```python
from build123d import *

# Parameters (mm, degrees)
SKETCH2_W                = 100
SKETCH2_H                = 100
BOSS_EXTRUDE1_DEPTH      = 5
SKETCH3_R                = 19.95
BOSS_EXTRUDE2_DEPTH      = 60
SKETCH4_R                = 5
CUT_EXTRUDE1_DEPTH       = 43.5
SKETCH10_R               = 1
SKETCH11_R               = 1
SKETCH15_R               = 5
BOSS_EXTRUDE3_DEPTH      = 10
BOSS_EXTRUDE3_DEPTH_BACK = 2
SKETCH18_R               = 5
BOSS_EXTRUDE4_DEPTH      = 1
SKETCH19_R               = 2.7
CUT_EXTRUDE3_DEPTH       = 36
SKETCH20_R               = 0.75
CUT_REVOLVE4_ANGLE       = 180
SKETCH21_W               = 20
SKETCH21_H               = 20
CUT_EXTRUDE4_DEPTH       = 2
SKETCH23_R               = 1.5
BOSS_EXTRUDE5_DEPTH      = 5


with BuildPart() as part:
    # Sketch2 → Boss-Extrude1 (new body)
    with BuildSketch(Plane(origin=(0, 0, 0), x_dir=(1, 0, 0), z_dir=(0, 1, 0))):
        with Locations((-25, 0)):
            Rectangle(SKETCH2_W, SKETCH2_H)
    extrude(amount=BOSS_EXTRUDE1_DEPTH)

    # Sketch3 → Boss-Extrude2 (add)
    with BuildSketch(Plane(origin=(0, 5, 0), x_dir=(1, 0, 0), z_dir=(0, 1, 0))):
        Circle(SKETCH3_R)
    extrude(amount=BOSS_EXTRUDE2_DEPTH)

    # Sketch4 → Cut-Extrude1 (cut)
    with BuildSketch(Plane(origin=(0, 65, 0), x_dir=(1, 0, 0), z_dir=(0, 1, 0))):
        Circle(SKETCH4_R)
    extrude(amount=-CUT_EXTRUDE1_DEPTH, mode=Mode.SUBTRACT)

    # Sketch10 → Cut-Revolve2 (revolve, cut)
    with BuildSketch(Plane.XY):
        with Locations((19.95, 6)):
            Circle(SKETCH10_R)
    revolve(axis=Axis((0, 0, 0), (0, 1, 0)), mode=Mode.SUBTRACT)

    # Sketch11 → Cut-Revolve3 (revolve, cut)
    with BuildSketch(Plane.XY):
        with Locations((19.95, 53)):
            Circle(SKETCH11_R)
    revolve(axis=Axis((0, 0, 0), (0, 1, 0)), mode=Mode.SUBTRACT)

    # Sketch15 → Boss-Extrude3 (add, two sides)
    with BuildSketch(Plane(origin=(0, 38, 0), x_dir=(1, 0, 0), z_dir=(0, 1, 0))) as boss_extrude3_sk:
        Circle(SKETCH15_R)
    extrude(amount=BOSS_EXTRUDE3_DEPTH)
    extrude(boss_extrude3_sk.sketch, amount=-BOSS_EXTRUDE3_DEPTH_BACK)

    # Sketch18 → Boss-Extrude4 (add)
    with BuildSketch(Plane(origin=(0, 65, 0), x_dir=(1, 0, 0), z_dir=(0, 1, 0))):
        Circle(SKETCH18_R)
    extrude(amount=-BOSS_EXTRUDE4_DEPTH)

    # Sketch19 → Cut-Extrude3 (cut)
    with BuildSketch(Plane(origin=(0, 65, 0), x_dir=(1, 0, 0), z_dir=(0, 1, 0))):
        Circle(SKETCH19_R)
    extrude(amount=-CUT_EXTRUDE3_DEPTH, mode=Mode.SUBTRACT)

    # Sketch20 → Cut-Revolve4 (revolve, cut)
    with BuildSketch(Plane(origin=(0, 0, 0), x_dir=(0, 0, -1), z_dir=(1, 0, 0))):
        with Locations((-19.95, 29)):
            Circle(SKETCH20_R)
    revolve(axis=Axis((0, 0, 0), (0, 1, 0)), revolution_arc=CUT_REVOLVE4_ANGLE, mode=Mode.SUBTRACT)

    # Sketch21 → Cut-Extrude4 (cut)
    with BuildSketch(Plane(origin=(0, 65, 0), x_dir=(1, 0, 0), z_dir=(0, 1, 0))):
        Rectangle(SKETCH21_W, SKETCH21_H)
    extrude(amount=-CUT_EXTRUDE4_DEPTH, mode=Mode.SUBTRACT)

    # Sketch23 → Boss-Extrude5 (add)
    with BuildSketch(Plane(origin=(0, 65, 0), x_dir=(1, 0, 0), z_dir=(0, 1, 0))):
        with Locations((0, -15)):
            Circle(SKETCH23_R)
        with Locations((0, 15)):
            Circle(SKETCH23_R)
        with Locations((-15, 0)):
            Circle(SKETCH23_R)
        with Locations((15, 0)):
            Circle(SKETCH23_R)
    extrude(amount=BOSS_EXTRUDE5_DEPTH)


solid = part.part
```
Here's how the part is built. I have some questions about the finished solid (model axes, mm). A direction names the side the tool comes from. Coordinates: 2 decimals unless noted, no trailing zeros. Write each loop counter-clockwise with the first axis right and the second up, starting at its lowest first coordinate (ties: lowest second). Pieces come first, ordered by that corner, then holes. Notation, with made-up numbers: (45.5, 87.5) -> (81.5, 87.5) arc R21 cw to (81.5, 102.5) -> close; hole circle Ø9 at (-16.5, 3). An arc over 180 degrees is marked (long way). Use a Markdown table: item, result. Add a question column.
(1) For faces 1 (the cylindrical face through (13.5, 67.46, -0.07)), 2 (the flat face through (-15, 70, 0)), 3 (the flat face through (0, 21.5, 0)), which set-ups out of +Z, -Z, +X, -X, +Y, -Y let a thin tool reach every point of the face, with its end or its side?
(2) I'm going to push flat-ended pins straight in: P1, Ø22, axis at x = -2.5, z = 2, coming from the +Y side; P2, Ø1.5, axis at y = 53, z = 14, coming from the -X side; P3, Ø1, axis at x = 5, y = 64, coming from the +Z side; P4, Ø3, axis at x = -0.5, z = 2.5, coming from the -Y side. Where does each tip first touch, or does it pass through?
(3) If we section it at B-B, the plane z = -31.5: Write out the boundary of the cut face in (x, y), and give its area (3 significant figures).
(4) If we section it at A-A, the plane y = 45: Write out the boundary of the cut face in (x, z).
(5) If we section it at D-D, the plane y = 18.5: Write out the boundary of the cut face in (x, z), and give its area (3 significant figures).
(6) If we section it at C-C, the plane x = -59.5: Write out the boundary of the cut face in (y, z), and give its area (3 significant figures).
(7) We'd pull the mould along Z, two halves only. Please class faces 4 (the cylindrical face through (-0.325, 67.465, 16.464)), 5 (the cylindrical face through (-1.08, 55.6, 4.88)), 6 (the flat face through (0, 70, -15)), 7 (the cylindrical face through (19.03, 59.42, -5.99)): +Z half, -Z half, draft (parallel to the pull), parting line (faces both ways), or undercut.
(8) Please list where these lines run through material, in increasing order: line 1 (X direction, y = 45, z = 0); line 2 (X direction, y = 28, z = 0); line 3 (Y direction, x = -16, z = -42.5).
Outcome:
| question | item | result |
|---|---|---|
| 1 | face 1 | +Y |
| 1 | face 2 | +Z, -Z, +X, -X, +Y |
| 1 | face 3 | none |
| 2 | P1 | stops at y = 65 |
| 2 | P2 | stops at x = -13.55 |
| 2 | P3 | stops at z = 19.44 |
| 2 | P4 | stops at y = 0 |
| 3 | outline | (-75, 0) -> (25, 0) -> (25, 5) -> (-75, 5) -> close |
| 3 | area | 500 mm^2 |
| 4 | outline | circle Ø39.9 at (0, 0); hole circle Ø5.4 at (0, 0) |
| 5 | outline | circle Ø39.9 at (0, 0) |
| 5 | area | 1,250 mm^2 |
| 6 | outline | (0, -50) -> (5, -50) -> (5, 50) -> (0, 50) -> close |
| 6 | area | 500 mm^2 |
| 7 | face 4 | undercut |
| 7 | face 5 | undercut |
| 7 | face 6 | draft |
| 7 | face 7 | parting line |
| 8 | line 1 | x = -19.95 to -2.7, 2.7 to 19.95 |
| 8 | line 2 | x = -19.95 to -5, 5 to 19.95 |
| 8 | line 3 | y = 0 to 5 |
